from build123d import *

# Parameters (mm, degrees)
F0_W      = 1
F0_H      = 7
F1_DEPTH  = 25.5
F2_W      = 1
F2_H      = 7
F3_DEPTH  = 3
F4_W      = 1
F4_H      = 7
F5_DEPTH  = 3
F7_DEPTH  = 1
F9_DEPTH  = 1
F13_D     = 5
F13_DEPTH = 6
F13_TIP   = 1.5021515476


# Not quite as in the source:
# - a pattern or mirror of a feature is missing from the dataset's text; its kind, count and spacing are read off the source's solid


with BuildPart() as f1:
    # F0 (on Front) → F1 (new body, symmetric)
    with BuildSketch(Plane.XZ):
        with BuildLine():
            ThreePointArc((1.8823727184, 19.4089328132), (19.4772198973, -0.9422871488), (0, -19.5))
            Line((0, -19.5), (0, -20.5))
            ThreePointArc((0, -20.5), (20.4490247642, -1.444778942), (2.8823727184, 20.2963525667))
            Line((2.8823727184, 20.2963525667), (2.8823727184, 21.2562642992))
            Line((2.8823727184, 21.2562642992), (2.8823727184, 28.2562642992))
            Line((2.8823727184, 28.2562642992), (2.8823727184, 29.5688871337))
            Line((2.8823727184, 29.5688871337), (6.8823727184, 29.5688871337))
            Line((6.8823727184, 29.5688871337), (6.8823727184, 34.5688871337))
            Line((6.8823727184, 34.5688871337), (3.8823727184, 34.5688871337))
            Line((3.8823727184, 34.5688871337), (3.8823727184, 33.5702374578))
            Line((3.8823727184, 33.5702374578), (3.8823727184, 33.5688871337))
            Line((3.8823727184, 33.5688871337), (5.8823727184, 33.5688871337))
            Line((5.8823727184, 33.5688871337), (5.8823727184, 30.5688871337))
            Line((5.8823727184, 30.5688871337), (1.8823727184, 30.5688871337))
            Line((1.8823727184, 30.5688871337), (1.8823727184, 20.578497021))
            Line((1.8823727184, 20.578497021), (1.8823727184, 19.4089328132))
        make_face()
        Polygon((0, 20.561426878), (1.8823727184, 20.578497021), (1.8823727184, 30.5688871337), (5.8823727184, 30.5688871337), (5.8823727184, 33.5688871337), (3.8823727184, 33.5688871337), (3.8823727184, 33.5702374578), (0, 33.5702374578), align=None)
        with Locations((3.3823727184, 24.7562642992)):
            Rectangle(F0_W, F0_H)
        Polygon((3.8823727184, 28.2562642992), (3.8823727184, 21.2562642992), (3.8823727184, 20.6377897412), (10.0385518745, 20.6377897412), (10.0385518745, 28.6377897412), (3.8823727184, 28.6377897412), align=None)
    extrude(amount=F1_DEPTH, both=True)

    # F2 (on face) → F3 (cut)
    with BuildSketch(Plane.XZ.offset(25.5)):
        with Locations((3.3823727184, 24.7562642992)):
            Rectangle(F2_W, F2_H)
    extrude(amount=-F3_DEPTH, mode=Mode.SUBTRACT)

    # F4 (on face) → F5 (cut)
    with BuildSketch(Plane(origin=(0, 25.5, 0), x_dir=(-1, 0, 0), z_dir=(0, 1, 0))):
        with Locations((-3.3823727184, 24.7562642992)):
            Rectangle(F4_W, F4_H)
    extrude(amount=-F5_DEPTH, mode=Mode.SUBTRACT)

    # F6 (on face) → F7 (cut)
    with BuildSketch(Plane.XZ.offset(25.5)):
        Polygon((0, 20.561426878), (1.8823727184, 20.578497021), (1.8823727184, 30.5688871337), (5.8823727184, 30.5688871337), (5.8823727184, 33.5688871337), (3.8823727184, 33.5688871337), (3.8823727184, 33.5702374578), (0, 33.5702374578), align=None)
    extrude(amount=-F7_DEPTH, mode=Mode.SUBTRACT)

    # F8 (on face) → F9 (cut)
    with BuildSketch(Plane(origin=(0, 25.5, 0), x_dir=(-1, 0, 0), z_dir=(0, 1, 0))):
        Polygon((-1.8823727184, 30.5688871337), (-1.8823727184, 20.578497021), (0, 20.561426878), (0, 33.5702374578), (-3.8823727184, 33.5702374578), (-3.8823727184, 33.5688871337), (-5.8823727184, 33.5688871337), (-5.8823727184, 30.5688871337), align=None)
    extrude(amount=-F9_DEPTH, mode=Mode.SUBTRACT)

    # F10: F1 across plane


with BuildPart() as f1_1:
    add(f1.part)
    add(f1.part.mirror(Plane.YZ))

    # F13
    with Locations(Plane(origin=(-20.5, 0, 0), x_dir=(0, 1, 0), z_dir=(-1, 0, 0))):
        with Locations((13.9512377791, 0)):
            f13 = Hole(F13_D / 2, depth=F13_DEPTH)
            with Locations((0, 0, -(F13_DEPTH + F13_TIP / 2))):  # 118° drill point
                Cone(0, F13_D / 2, F13_TIP, mode=Mode.SUBTRACT)

    # F13_copies: F13 across plane
    add(f13.mirror(Plane(origin=(-1.9e-05, 0, 0), x_dir=(0, 0, 1), z_dir=(1, 0, 0))), mode=Mode.SUBTRACT)


solid = f1_1.part
CAD build for the part. Positions are in the model's coordinates, mm. A direction names the side the tool comes from. Give positions to 0.01 mm unless a question says otherwise; leave off trailing zeros. Write each loop counter-clockwise with the first axis right and the second up, starting at its lowest first coordinate (ties: lowest second). Pieces come first, ordered by that corner, then holes. Notation, with made-up numbers: (-8.5, -31) -> (-2.5, -31) arc R21 ccw to (-2.5, -7) -> close; hole circle Ø10 at (45.25, 10.5). An arc over 180 degrees is marked (long way). Return JSON: item names as keys, results as strings.
Item 1: Drill centre lines: probe 1 along X at (y, z) = (23, 27.5); probe 2 along Z at (x, y) = (-10, -21.5); probe 3 along Z at (x, y) = (-4.5, 23). Where is each one in solid material? Low to high.
Answer below:
{"probe 1": "x = -10.04 to -3.88, -2.88 to 2.88, 3.88 to 10.04", "probe 2": "z = -17.9 to -16.74, 16.74 to 17.9, 20.64 to 28.64", "probe 3": "z = -20 to -18.97, 18.97 to 20, 20.64 to 28.64, 29.57 to 34.57"}
Item 2: Band-saw the part on A-A (z = 0). List the corners of the cut face in (x, y), then the cut area to 3 significant figures.
Answer below:
{"outline": "(-20.5, -25.5) -> (-19.5, -25.5) -> (-19.5, 11.45) -> (-20.5, 11.45) -> close; (-20.5, 16.45) -> (-19.5, 16.45) -> (-19.5, 25.5) -> (-20.5, 25.5) -> close; (19.5, -25.5) -> (20.5, -25.5) -> (20.5, 11.45) -> (19.5, 11.45) -> close; (19.5, 16.45) -> (20.5, 16.45) -> (20.5, 25.5) -> (19.5, 25.5) -> close", "area": "92.0 mm2"}
Item 3: Tool access for faces 5 (the flat face through (0, 0, 33.57)), 6 (the flat face through (3.882, 0, 21)), 7 (the flat face through (-7, 0, 20.638)), 8 (the flat face through (7, 0, 20.638)): list every direction of +Z, -Z, +X, -X, +Y, -Y with a clear straight run to the whole face (end or side of a thin tool).
Answer below:
{"face 5": "+Z, +Y, -Y", "face 6": "none", "face 7": "-X, +Y, -Y", "face 8": "+X, +Y, -Y"}
Item 4: Two-plate mould, pull along X, no slides. Class faces 1 (the flat face through (-7, 25.5, 25)), 2 (the flat face through (-6.882, 0, 32)), 3 (the flat face through (1.882, -6, 20)), 4 (the flat face through (6.882, 0, 32)): +X half, -X half, draft (parallel to the pull), parting line (faces both ways), or undercut.
Answer below:
{"face 1": "draft", "face 2": "-X half", "face 3": "undercut", "face 4": "+X half"}
Item 5: Drop flat-ended pins along their axis: pin 1 (0.5 mm diameter, centred on x = -3.5, y = 5.5, fed in from +Z); pin 2 (2 mm diameter, centred on x = 4, y = 6, fed in from -Z); pin 3 (2 mm diameter, centred on y = 4.5, z = -11, fed in from +X). Give the stop position or say it passes through.
Answer below:
{"pin 1": "stops at z = 33.57", "pin 2": "stops at z = -20.28", "pin 3": "stops at x = 17.9"}
Item 6: Band-saw the part on B-B (x = 18.5). List the corners of the cut face in (y, z).
Answer below:
{"outline": "(-25.5, -8.83) -> (25.5, -8.83) -> (25.5, -6.16) -> (-25.5, -6.16) -> close; (-25.5, 6.16) -> (25.5, 6.16) -> (25.5, 8.83) -> (-25.5, 8.83) -> close"}
Item 7: Band-saw the part on C-C (z = 13). List the corners of the cut face in (x, y).
Answer below:
{"outline": "(-15.85, -25.5) -> (-14.53, -25.5) -> (-14.53, 25.5) -> (-15.85, 25.5) -> close; (14.53, -25.5) -> (15.85, -25.5) -> (15.85, 25.5) -> (14.53, 25.5) -> close"}
